from build123d import *

# Parameters (mm, degrees)
BASE_FLANGE1_START                    = -3
BASE_FLANGE1_OUTLINE_W                = 88
BASE_FLANGE1_OUTLINE_H                = 300
BASE_FLANGE1_DEPTH                    = 3
CUT_EXTRUDE2_DEPTH                    = 509.426019398
CUT_EXTRUDE2_DEPTH_BACK               = 3
SKETCH14_OUTSIDE_W                    = 152.53
SKETCH14_OUTSIDE_H                    = 364.53
T_LE_PLI_E_SUR_AR_TE2_STRIP_W         = 13.4732
T_LE_PLI_E_SUR_AR_TE2_STRIP_H         = 3
T_LE_PLI_E_SUR_AR_TE2_STRIP_CUT_DEPTH = 88
T_LE_PLI_E_SUR_AR_TE2_DEPTH           = 88
D_GAGEMENT_M51_D                      = 5.5
T_LE_PLI_E_SUR_AR_TE3_STRIP_W         = 13.4732
T_LE_PLI_E_SUR_AR_TE3_STRIP_H         = 3
T_LE_PLI_E_SUR_AR_TE3_STRIP_CUT_DEPTH = 74
T_LE_PLI_E_SUR_AR_TE3_DEPTH           = 74
T_LE_PLI_E_SUR_AR_TE3_PROFILE_W       = 88
T_LE_PLI_E_SUR_AR_TE3_PROFILE_H       = 199.2634
T_LE_PLI_E_SUR_AR_TE3_FLAT_DEPTH      = 3
BOSS_EXTRUDE2_DEPTH                   = 154
CUT_EXTRUDE3_REACH                    = 544.8
SKETCH48_W                            = 41
SKETCH48_H                            = 21
BOSS_EXTRUDE3_REACH                   = 548.341
CUT_EXTRUDE4_REACH                    = 544.8
SKETCH50_R                            = 2


# Read off the part's stored shape, not the designer's step: Base-Flange1
# Sheet-metal steps are written as plain solids
with BuildPart() as part:
    # Base-Flange1 outline → Base-Flange1 (new body)
    with BuildSketch(Plane(origin=(0, 0, 0), x_dir=(1, 0, 0), z_dir=(0, 1, 0)).offset(BASE_FLANGE1_START)):
        with Locations((48.130435799, 350)):
            Rectangle(BASE_FLANGE1_OUTLINE_W, BASE_FLANGE1_OUTLINE_H)
    extrude(amount=BASE_FLANGE1_DEPTH)

    # Sketch14 outside → Cut-Extrude2 (cut, two sides: drawn at the far end of the back side and taken through both)
    with BuildSketch(Plane.XZ.offset(3).offset(-CUT_EXTRUDE2_DEPTH_BACK)):
        with Locations((48.13, -350)):
            Rectangle(SKETCH14_OUTSIDE_W, SKETCH14_OUTSIDE_H)
        with BuildLine():
            Line((85.130435799, -200), (11.130435799, -200))
            Line((11.130435799, -200), (11.130435799, -213))
            Line((11.130435799, -213), (21.130435799, -213))
            Line((21.130435799, -213), (21.130435799, -302))
            Line((21.130435799, -302), (11.130435799, -302))
            Line((11.130435799, -302), (11.130435799, -315))
            Line((11.130435799, -315), (21.130435799, -315))
            Line((21.130435799, -315), (37.130435799, -331))
            ThreePointArc((37.130435799, -331), (32.754046891, -352.5), (37.130435799, -374))
            ThreePointArc((37.130435799, -374), (29.130435799, -382), (37.130435799, -390))
            Line((37.130435799, -390), (4.130435799, -390))
            Line((4.130435799, -390), (4.130435799, -500))
            Line((4.130435799, -500), (92.130435799, -500))
            Line((92.130435799, -500), (92.130435799, -390))
            Line((92.130435799, -390), (59.130435799, -390))
            ThreePointArc((59.130435799, -390), (67.130435799, -382), (59.130435799, -374))
            ThreePointArc((59.130435799, -374), (63.506824707, -352.5), (59.130435799, -331))
            Line((59.130435799, -331), (75.130435799, -315))
            Line((75.130435799, -315), (85.130435799, -315))
            Line((85.130435799, -315), (85.130435799, -302))
            Line((85.130435799, -302), (75.130435799, -302))
            Line((75.130435799, -302), (75.130435799, -213))
            Line((75.130435799, -213), (85.130435799, -213))
            Line((85.130435799, -213), (85.130435799, -200))
        make_face(mode=Mode.SUBTRACT)
    extrude(amount=CUT_EXTRUDE2_DEPTH + CUT_EXTRUDE2_DEPTH_BACK, mode=Mode.SUBTRACT)

    # Tôle pliée sur arête2 strip (across the edge) → Tôle pliée sur arête2 strip cut (cut)
    with BuildSketch(Plane(origin=(92.130435799, 0, -500), x_dir=(0, 0, 1), z_dir=(-1, 0, 0))):
        with Locations((-3, -1.5)):
            Rectangle(T_LE_PLI_E_SUR_AR_TE2_STRIP_W, T_LE_PLI_E_SUR_AR_TE2_STRIP_H)
    extrude(amount=T_LE_PLI_E_SUR_AR_TE2_STRIP_CUT_DEPTH, mode=Mode.SUBTRACT)

    # Tôle pliée sur arête2 section (across the edge) → Tôle pliée sur arête2 (add)
    with BuildSketch(Plane(origin=(92.130435799, 0, -500), x_dir=(0, 0, 1), z_dir=(-1, 0, 0))):
        with BuildLine():
            Line((0, 0.7366), (0, 66.5))
            Line((0, 66.5), (3, 66.5))
            Line((3, 66.5), (3, 0.7366))
            ThreePointArc((3, 0.7366), (3.215745145, 0.215745145), (3.7366, 0))
            Line((3.7366, 0), (3.7366, -3))
            ThreePointArc((3.7366, -3), (1.094424801, -1.905575199), (0, 0.7366))
        make_face()
    extrude(amount=T_LE_PLI_E_SUR_AR_TE2_DEPTH)

    # Dégagement M51 (through all)
    with Locations(Plane(origin=(58.130435799, 53.6, -500), x_dir=(-1, 0, 0), z_dir=(0, 0, -1))):
        with Locations((0, 0), (20, 0), (0, -39.7), (20, -39.7)):
            Hole(D_GAGEMENT_M51_D / 2)

    # Tôle pliée sur arête3 strip (across the edge) → Tôle pliée sur arête3 strip cut (cut)
    with BuildSketch(Plane(origin=(11.130435799, 0, -200), x_dir=(0, 0, -1), z_dir=(1, 0, 0))):
        with Locations((-3, -1.5)):
            Rectangle(T_LE_PLI_E_SUR_AR_TE3_STRIP_W, T_LE_PLI_E_SUR_AR_TE3_STRIP_H)
    extrude(amount=T_LE_PLI_E_SUR_AR_TE3_STRIP_CUT_DEPTH, mode=Mode.SUBTRACT)

    # Tôle pliée sur arête3 bend section (across the edge) → Tôle pliée sur arête3 (add)
    with BuildSketch(Plane(origin=(11.130435799, 0, -200), x_dir=(0, 0, -1), z_dir=(1, 0, 0))):
        with BuildLine():
            Line((0, 0.7366), (3, 0.7366))
            ThreePointArc((3, 0.7366), (3.215745145, 0.215745145), (3.7366, 0))
            Line((3.7366, 0), (3.7366, -3))
            ThreePointArc((3.7366, -3), (1.094424801, -1.905575199), (0, 0.7366))
        make_face()
    extrude(amount=T_LE_PLI_E_SUR_AR_TE3_DEPTH)

    # Tôle pliée sur arête3 profile (on flange) → Tôle pliée sur arête3 flat (add)
    with BuildSketch(Plane(origin=(0, 0, -200), x_dir=(-1, 0, 0), z_dir=(0, 0, -1))):
        with Locations((-48.130435799, 100.3683)):
            Rectangle(T_LE_PLI_E_SUR_AR_TE3_PROFILE_W, T_LE_PLI_E_SUR_AR_TE3_PROFILE_H)
    extrude(amount=T_LE_PLI_E_SUR_AR_TE3_FLAT_DEPTH)

    # Sketch47 → Boss-Extrude2 (add)
    with BuildSketch(Plane(origin=(0, 0, -203), x_dir=(-1, 0, 0), z_dir=(0, 0, -1))):
        Polygon((-72.190435799, 83.5), (-72.190435799, 110.5), (-92.130435799, 110.5), (-92.130435799, 107.5), (-75.190435799, 107.5), (-75.190435799, 86.5), (-92.130435799, 86.5), (-92.130435799, 83.5), align=None)
    extrude(amount=BOSS_EXTRUDE2_DEPTH)

    # Sketch48 → Cut-Extrude3 (cut, up to next)
    with BuildSketch(Plane.ZY.offset(-72.190435799), mode=Mode.PRIVATE) as cut_extrude3_sk1:
        with Locations((-328.97, 97)):
            Rectangle(SKETCH48_W, SKETCH48_H)
    cut_extrude3_tool1 = extrude(cut_extrude3_sk1.sketch, amount=-CUT_EXTRUDE3_REACH, mode=Mode.PRIVATE) & part.part
    add(cut_extrude3_tool1.solids().sort_by_distance((72.190436, 97, -328.97))[0], mode=Mode.SUBTRACT)

    # Sketch49 → Boss-Extrude3 (add, up to next)
    with BuildSketch(Plane(origin=(0, 0, 0), x_dir=(1, 0, 0), z_dir=(0, 1, 0)), mode=Mode.PRIVATE) as boss_extrude3_sk1:
        Polygon((75.130435799, 315), (85.130435799, 315), (85.130435799, 302), (75.130435799, 302), (75.130435799, 304), (83.130435799, 304), (83.130435799, 313), (75.130435799, 313), align=None)
    boss_extrude3_tool1 = extrude(boss_extrude3_sk1.sketch, amount=BOSS_EXTRUDE3_REACH, mode=Mode.PRIVATE) - part.part
    add(boss_extrude3_tool1.solids().sort_by_distance((80.130436, 0, -314.835988))[0])

    # Sketch50 → Cut-Extrude4 (cut, up to next)
    with BuildSketch(Plane.ZY.offset(-72.190435799), mode=Mode.PRIVATE) as cut_extrude4_sk1:
        with Locations((-352.22, 102)):
            Circle(SKETCH50_R)
    cut_extrude4_tool1 = extrude(cut_extrude4_sk1.sketch, amount=-CUT_EXTRUDE4_REACH, mode=Mode.PRIVATE) & part.part
    # Sketch50 → Cut-Extrude4 (cut, up to next)
    with BuildSketch(Plane.ZY.offset(-72.190435799), mode=Mode.PRIVATE) as cut_extrude4_sk2:
        with Locations((-352.22, 92)):
            Circle(SKETCH50_R)
    cut_extrude4_tool2 = extrude(cut_extrude4_sk2.sketch, amount=-CUT_EXTRUDE4_REACH, mode=Mode.PRIVATE) & part.part
    # Sketch50 → Cut-Extrude4 (cut, up to next)
    with BuildSketch(Plane.ZY.offset(-72.190435799), mode=Mode.PRIVATE) as cut_extrude4_sk3:
        with Locations((-305.72, 102)):
            Circle(SKETCH50_R)
    cut_extrude4_tool3 = extrude(cut_extrude4_sk3.sketch, amount=-CUT_EXTRUDE4_REACH, mode=Mode.PRIVATE) & part.part
    # Sketch50 → Cut-Extrude4 (cut, up to next)
    with BuildSketch(Plane.ZY.offset(-72.190435799), mode=Mode.PRIVATE) as cut_extrude4_sk4:
        with Locations((-305.72, 92)):
            Circle(SKETCH50_R)
    cut_extrude4_tool4 = extrude(cut_extrude4_sk4.sketch, amount=-CUT_EXTRUDE4_REACH, mode=Mode.PRIVATE) & part.part
    add(cut_extrude4_tool1.solids().sort_by_distance((72.190436, 102, -352.22))[0], mode=Mode.SUBTRACT)
    add(cut_extrude4_tool2.solids().sort_by_distance((72.190436, 92, -352.22))[0], mode=Mode.SUBTRACT)
    add(cut_extrude4_tool3.solids().sort_by_distance((72.190436, 102, -305.72))[0], mode=Mode.SUBTRACT)
    add(cut_extrude4_tool4.solids().sort_by_distance((72.190436, 92, -305.72))[0], mode=Mode.SUBTRACT)


solid = part.part
Geometry check sheet. Reference: the model listing, model coordinates, mm. A direction names the side the tool comes from. Round coordinates to 2 decimals unless told otherwise and drop trailing zeros. Order: outer loops, then holes, each group sorted by start corner. A loop starts at its lowest first (then second) coordinate and runs counter-clockwise, first axis right, second up. Notation, with made-up numbers: (36, 61) -> (46, 61) arc R37 cw to (46, 98) -> close; hole circle Ø9 at (34.25, 83.5). An arc over 180 degrees is marked (long way). Use one line per item in the form item = value.
1. Cross-section at A-A, the plane y = 38.5. Enter the section's corners in (x, z), plus the area to 3 significant figures.
Working result:
outline = (4.13, -500) -> (92.13, -500) -> (92.13, -497) -> (4.13, -497) -> close; (4.13, -203) -> (92.13, -203) -> (92.13, -200) -> (4.13, -200) -> close; (75.13, -315) -> (85.13, -315) -> (85.13, -302) -> (75.13, -302) -> (75.13, -304) -> (83.13, -304) -> (83.13, -313) -> (75.13, -313) -> close
area = 586 mm^2
2. Cross-section at D-D, the plane z = -382. Enter the section's corners in (x, y).
Working result:
outline = (29.13, -3) -> (67.13, -3) -> (67.13, 0) -> (29.13, 0) -> close
3. Set-up check for faces 5 (the face through (84, 97, -203)), 6 (the face through (85.13, 40, -309)), 7 (the face through (49, 34, -497)), 8 (the face through (79, 41, -313)): record each of +Z, -Z, +X, -X, +Y, -Y from which the full face is reachable in a straight line by a thin tool's end or side.
Working result:
face_5 = -Z, +X
face_6 = +X, -Y
face_7 = +X, -X, +Y
face_8 = -X
4. Mould release check, pull along Y, two halves, no side actions. Record for faces 1 (the face through (75, 97, -357)), 2 (the face through (48, -3, -385)), 3 (the face through (79, 41, -304)), 4 (the face through (75.19, 97, -255)): pulls with the +Y half, pulls with the -Y half, needs draft (parallel to the pull), parting line crosses it, or undercut.
Working result:
face_1 = needs draft
face_2 = pulls with the -Y half
face_3 = undercut
face_4 = undercut
5. Cross-section at C-C, the plane x = 47. Enter the section's corners in (y, z).
Working result:
outline = (-3, -496.26) arc R3.74 ccw to (0.74, -500) -> (66.5, -500) -> (66.5, -497) -> (0.74, -497) arc R0.74 cw to (0, -496.26) -> (0, -203.74) arc R0.74 cw to (0.74, -203) -> (200, -203) -> (200, -200) -> (0.74, -200) arc R3.74 ccw to (-3, -203.74) -> close
6. Cross-section at B-B, the plane z = -220. Enter the section's corners in (x, y).
Working result:
outline = (21.13, -3) -> (75.13, -3) -> (75.13, 0) -> (21.13, 0) -> close; (72.19, 83.5) -> (92.13, 83.5) -> (92.13, 86.5) -> (75.19, 86.5) -> (75.19, 107.5) -> (92.13, 107.5) -> (92.13, 110.5) -> (72.19, 110.5) -> close
7. Scan lines: line 1 along Y through (x, z) = (74.65, -352.22); line 2 along Y through (x, z) = (73, -305.72); line 3 along X through (y, z) = (53, -498). Record each from-to range of solid material in increasing order. Write a range as from..to.
Working result:
line_1 = 83.5..90, 94..100, 104..110.5
line_2 = -3..0, 83.5..90, 94..100, 104..110.5
line_3 = 4.13..35.45, 40.81..55.45, 60.81..92.13
8. Go/stop test with flat-tipped pins: pin 1 (5 mm diameter, centred on y = 102, z = -305.72, fed in from +X); pin 2 (1.1 mm diameter, centred on y = -1, z = -206.5, fed in from -X); pin 3 (0.9 mm diameter, centred on x = 17, y = -1, fed in from -Z). Record where each tip stops, or that it passes through.
Working result:
pin_1 = 75.19
pin_2 = 11.13
pin_3 = -499.77
